Could you check a few things on this model? Use its own coordinates, in mm. A direction names the side the tool comes from. Round coordinates to 2 decimals unless told otherwise and drop trailing zeros. Order: outer loops, then holes, each group sorted by start corner. A loop starts at its lowest first (then second) coordinate and runs counter-clockwise, first axis right, second up. Notation, with made-up numbers: (27.25, -30) - (32.25, -30) arc R14 cw to (32.25, -20) - close; hole circle Ø3 at (4, 60.25). An arc over 180 degrees is marked (long way). Use one line per item in the form item = value.
from build123d import *

# Parameters (mm, degrees)
CORTAR_EXTRUIR1_REACH   = 53.334
CROQUIS2_R              = 2
CROQUIS3_R              = 2
SALIENTE_EXTRUIR1_DEPTH = 6.6
CORTAR_EXTRUIR2_DEPTH   = 4.2


with BuildPart() as part:
    # Croquis1 → Revolución1 (revolve)
    with BuildSketch(Plane.XY, mode=Mode.PRIVATE) as revoluci_n1_sk:
        Polygon((-2.5, 7.5), (-2.5, 0), (4.9, 0), (4.9, 7.5), (2.5, 7.5), (2.5, 25.5), (19.5, 25.5), (19.5, 26), (24, 26), (24, 30), (22.5, 30), (22.5, 27.5), (19.5, 27.5), (19.5, 30), (18.5, 30), (18.5, 27), (-18.5, 27), (-18.5, 30), (-19.5, 30), (-19.5, 27.5), (-22.5, 27.5), (-22.5, 30), (-24, 30), (-24, 26), (-19.5, 26), (-19.5, 25.5), (-2.5, 25.5), align=None)
    revolve(revoluci_n1_sk.sketch.rotate(Axis((-2.5, 0, 0), (1, 0, 0)), 180), axis=Axis((-2.5, 0, 0), (1, 0, 0)))

    # Croquis2 → Cortar-Extruir1 (cut, up to next)
    with BuildSketch(Plane(origin=(4.9, 0, 0), x_dir=(0, 0, -1), z_dir=(1, 0, 0)), mode=Mode.PRIVATE) as cortar_extruir1_sk1:
        with Locations(Location((0, 0, 0), (0, 0, 90))):
            Circle(CROQUIS2_R)
    cortar_extruir1_tool1 = extrude(cortar_extruir1_sk1.sketch, amount=-CORTAR_EXTRUIR1_REACH, mode=Mode.PRIVATE) & part.part
    add(cortar_extruir1_tool1.solids().sort_by_distance((4.9, 0, 0))[0], mode=Mode.SUBTRACT)

    # Croquis3 → Saliente-Extruir1 (add)
    with BuildSketch(Plane.ZY.offset(2.5)):
        Polygon((0, 8.256108849), (-7.15, 4.128054425), (-7.15, -4.128054425), (0, -8.256108849), (7.15, -4.128054425), (7.15, 4.128054425), align=None)
        with Locations(Location((0, 0, 0), (0, 0, 90))):
            Circle(CROQUIS3_R, mode=Mode.SUBTRACT)
    extrude(amount=SALIENTE_EXTRUIR1_DEPTH)

    # Croquis4 → Cortar-Extruir2 (cut)
    with BuildSketch(Plane.ZY.offset(9.1)):
        Polygon((6.15, 3.550704156), (0, 7.101408311), (-6.15, 3.550704156), (-6.15, -3.550704156), (0, -7.101408311), (6.15, -3.550704156), align=None)
    extrude(amount=-CORTAR_EXTRUIR2_DEPTH, mode=Mode.SUBTRACT)


solid = part.part
Item 1: Will these pins go through, and if not, where does the flat tip stop? P1, Ø6, axis at y = -4, z = 15, coming from the +X side; P2, Ø15.5, axis at y = -1, z = 1, coming from the -X side; P3, Ø3.5, axis at x = -7.5, y = -1.5, coming from the +Z side; P4, Ø3, axis at y = 0, z = 0, coming from the -X side.
Found:
P1 = 2.5
P2 = -9.1
P3 = 27
P4 = through
Item 2: For faces 1 (the face through (2.5, 5, -6)), 2 (the face through (-5.75, 6.16, 3.63)), 3 (the face through (-24, 9, -25)), 4 (the face through (-18.5, -25, -11)), which set-ups out of +Z, -Z, +X, -X, +Y, -Y let a thin tool reach every point of the face, with its end or its side?
Found:
face_1 = +X
face_2 = -X
face_3 = +Z, -Z, -X, +Y, -Y
face_4 = none
Item 3: If we mould it in two halves opening along X, with no side actions, what happens to faces 5 (the face through (24, -9, -25)), 6 (the face through (-21.021, -12.69, 24.397)), 7 (the face through (-19.007, -16.128, -25.296))? For each: released by +X, released by -X, zero draft, split by the parting line, or undercut.
Found:
face_5 = released by +X
face_6 = undercut
face_7 = zero draft
Item 4: Imagine slicing it at A-A on x = 8. Please give me the cut outline in (y, z).
Found:
outline = circle Ø54 at (0, 0); hole circle Ø51 at (0, 0)
Item 5: I need wall thicknesses on L1, parallel to Z at x = -8, y = 0; L2, parallel to Z at x = -10, y = 0; L3, parallel to Z at x = -21.2, y = 0. Which ranges of each line are inside material? Lowest first, please.
Found:
L1 = -27 to -25.5, -7.15 to -6.15, 6.15 to 7.15, 25.5 to 27
L2 = -27 to -25.5, 25.5 to 27
L3 = -27.5 to -26, 26 to 27.5
